Autodesk Inventor part; units mm, degrees
ref_plane "YZ Plane" through (0, 0, 0) normal (1, 0, 0) x (0, 1, 0)
ref_plane "XZ Plane" through (0, 0, 0) normal (0, 1, 0) x (-1, 0, 0)
ref_plane "XY Plane" through (0, 0, 0) normal (0, 0, 1) x (1, 0, 0)
sketch "Sketch1" plane through (0, 0, 0) normal (0, 0, 1) x (1, 0, 0)
  line L0 (-11.7577, -18.2929) -> (28.2423, -18.2929)
  line L1 (28.2423, -18.2929) -> (28.2423, -3.2929)
  line L2 (28.2423, -3.2929) -> (-11.7577, -3.2929)
  line L3 (-11.7577, -3.2929) -> (-11.7577, -18.2929)
  point P0 (0, 0)
  dimension "d0" = 40
  dimension "d1" = 15
extrude "Extrusion1" add sketch "Sketch1" along normal blind 6
sketch "Sketch2" plane through (0, 0, 6) normal (0, 0, 1) x (1, 0, 0)
  line L0 (28.2423, -3.2929) -> (-11.7577, -3.2929)
  line L1 (15.2423, -3.2929) -> (15.2423, -18.2929)
  line L2 (1.2423, -3.2929) -> (1.2423, -18.2929)
  line L3 (-11.7577, -18.2929) -> (28.2423, -18.2929)
  line L4 (15.2423, -6.7382) -> (28.2423, -6.7382) construction
  line L5 (28.2423, -18.2929) -> (28.2423, -3.2929)
  line L6 (1.2423, -6.7382) -> (-11.7577, -6.7382) construction
  line L7 (-11.7577, -3.2929) -> (-11.7577, -18.2929)
  point P0 (0, 0)
  dimension "d4" = 14
extrude "Extrusion2" add sketch "Sketch2" along normal blind 25 contours L1 L3 L2 L0
sketch "Sketch4" plane through (0, 0, 6) normal (0, 0, 1) x (1, 0, 0)
  circle A0 centre (21.7423, -10.7929) radius 2.125
  line L0 (21.7423, -10.7929) -> (21.7423, -3.2929) construction
  line L1 (21.7423, -10.7929) -> (21.7423, -18.2929) construction
  line L2 (15.2423, -18.2929) -> (28.2423, -18.2929)
  line L3 (21.7423, -10.7929) -> (28.2423, -10.7929) construction
  line L4 (21.7423, -10.7929) -> (15.2423, -10.7929) construction
  line L5 (15.2423, -18.2929) -> (15.2423, -3.2929)
  line L6 (28.2423, -3.2929) -> (15.2423, -3.2929)
  line L7 (28.2423, -18.2929) -> (28.2423, -3.2929)
  circle A1 centre (-5.2577, -10.7929) radius 2.125
  line L8 (-5.2577, -10.7929) -> (-5.2577, -3.2929) construction
  line L9 (-5.2577, -10.7929) -> (-11.7577, -10.7929) construction
  line L10 (-11.7577, -3.2929) -> (-11.7577, -18.2929)
  line L11 (-5.2577, -10.7929) -> (-5.2577, -18.2929) construction
  line L12 (-5.2577, -10.7929) -> (1.2423, -10.7929) construction
  line L13 (1.2423, -3.2929) -> (1.2423, -18.2929)
  point P0 (0, 0)
  dimension "d12" = 4.25
  dimension "d13" = 4.25
extrude "Extrusion4" cut sketch "Sketch4" against normal up to next contours A0 | A1
sketch "Sketch5" plane through (1.2423, -18.2929, 6) normal (-1, 0, 0) x (0, 0, 1)
  circle A0 centre (10, 7.5) radius 4
  line L0 (10, 7.5) -> (10, 15) construction
  line L1 (10, 7.5) -> (10, 0) construction
  line L2 (-6, 15) -> (-6, 0)
  line L3 (13.9686, 7) -> (25, 7)
  line L4 (13.9686, 8) -> (25, 8)
  line L5 (25, 15) -> (25, 0)
  line L6 (27.4068, 8) -> (27.4068, 15) construction
  line L7 (27.4068, 7) -> (27.4068, 0) construction
  line L8 (0, 0) -> (25, 0)
  line L9 (0, 15) -> (25, 15)
  line L10 (10, 7.5) -> (10, 0) construction
  line L11 (0, 0) -> (25, 0)
  point P0 (-6, 18.2929)
  dimension "d16" = 8
  dimension "d17" = 16
  dimension "d18" = 1
extrude "Extrusion5" cut sketch "Sketch5" against normal up to next
sketch "Sketch6" plane through (-11.7577, -3.2929, 0) normal (0, 1, 0) x (1, 0, 0)
  circle A0 centre (20, -25) radius 2.125
  line L0 (27, -31) -> (13, -31)
  line L1 (20, -25) -> (27, -25) construction
  line L2 (20, -25) -> (13, -25) construction
  line L3 (27, -6) -> (27, -31)
  line L4 (13, -6) -> (13, -31)
  point P0 (11.7577, 0)
  dimension "d21" = 4.25
  dimension "d22" = 6
extrude "Extrusion6" cut sketch "Sketch6" against normal through all
properties part number "YRodClamp"
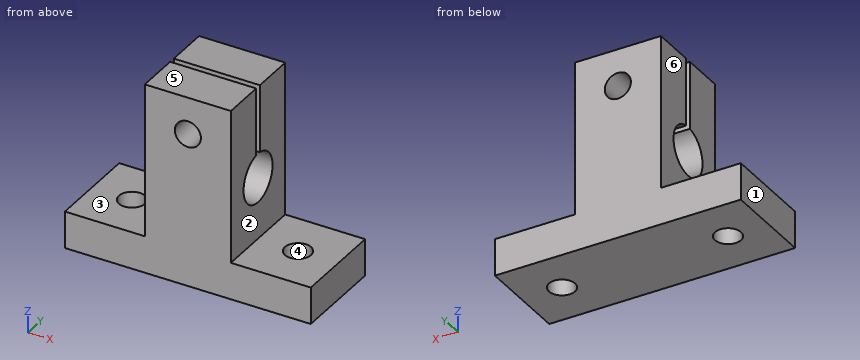
Source: CAD feature listing. Evaluate the final solid. Frame: model axes, mm. Face numbers are marked on the shaded views. A direction names the side the tool comes from. Round coordinates to 2 decimals unless told otherwise and drop trailing zeros. Loops run counter-clockwise (first coordinate to the right, second up) from the corner with the lowest first, then second, coordinate; pieces in that order, holes last.
Q1. Section D-D, the plane y = -17. Return loops of the section in (x, z) (3 decimals), plus the area to 3 significant figures.
Q2. Access query for the marked faces 1, 2 and 3. Directions: +Z, -Z, +X, -X, +Y, -Y. A direction counts if a zero-diameter tool reaches every point of the face in a straight line with its end or side. Return the directions, or none.
Q3. Section A-A, the plane z = 16. Return loops of the section in (x, y), plus the area to 3 significant figures.
Q4. Section C-C, the plane z = 25. Return loops of the section in (x, y), plus the area to 4 significant figures.
Q5. Ray query, line 1 (X direction, y = -13, z = 25); line 2 (Y direction, x = 5.25, z = 16); line 3 (Y direction, x = 6, z = 24). Return the intervals inside material, ascending.
Q6. Section B-B, the plane y = -7.5. Return loops of the section in (x, z) (3 decimals).
Q7. Mould query, pull axis X, two halves, no side actions, for the marked faces 4, 5 and 6. Classes: pulls with the +X half, pulls with the -X half, needs draft (parallel to the pull), parting line crosses it, or undercut.
Q8. First-contact query: P1, Ø7.5, axis at y = -10.5, z = 17, coming from the +X side; P2, Ø8, axis at x = 24, y = -10.5, coming from the +Z side; P3, Ø5, axis at y = -10.5, z = 13.5, coming from the -X side. Flat tips, straight axial feed; report the tip coordinate or a pass-through.
Solutions:
1. outline: (-11.758, 0) - (28.242, 0) - (28.242, 6) - (15.242, 6) - (15.242, 31) - (1.242, 31) - (1.242, 6) - (-11.758, 6) - close; hole circle Ø4.25 at (8.242, 25)
1. area: 576 mm2
2. face 1: +Z, -Z, -X, +Y, -Y
2. face 2: +Z, +X, +Y, -Y
2. face 3: +Z, -X, +Y, -Y
3. outline: (1.24, -18.29) - (15.24, -18.29) - (15.24, -14.79) - (1.24, -14.79) - close; (1.24, -6.79) - (15.24, -6.79) - (15.24, -3.29) - (1.24, -3.29) - close
3. area: 98.0 mm2
4. outline: (1.24, -18.29) - (6.12, -18.29) - (6.12, -11.29) - (1.24, -11.29) - close; (1.24, -10.29) - (6.12, -10.29) - (6.12, -3.29) - (1.24, -3.29) - close; (10.37, -18.29) - (15.24, -18.29) - (15.24, -11.29) - (10.37, -11.29) - close; (10.37, -10.29) - (15.24, -10.29) - (15.24, -3.29) - (10.37, -3.29) - close
4. area: 136.5 mm2
5. line 1: x = 1.24 to 6.12, 10.37 to 15.24
5. line 2: y = -18.29 to -14.79, -6.79 to -3.29
5. line 3: y = -18.29 to -11.29, -10.29 to -3.29
6. outline: (-11.758, 0) - (28.242, 0) - (28.242, 6) - (15.242, 6) - (15.242, 13.729) - (1.242, 13.729) - (1.242, 6) - (-11.758, 6) - close; (1.242, 18.271) - (15.242, 18.271) - (15.242, 31) - (1.242, 31) - close; hole circle Ø4.25 at (8.242, 25)
7. face 4: undercut
7. face 5: needs draft
7. face 6: pulls with the -X half
8. P1: stops at x = 15.24
8. P2: stops at z = 6
8. P3: stops at x = 1.24
